from build123d import *

# Parameters (mm, degrees)
BOSS_EXTRUDE1_DEPTH = 2.5
FILLET1_R           = 6
FILLET2_R           = 1.5
SKETCH3_R           = 0.9999999999999983
CUT_EXTRUDE1_DEPTH  = 3.5
BOSS_EXTRUDE2_DEPTH = 2.6
SKETCH5_R           = 2.9999999999999947
CUT_EXTRUDE2_DEPTH  = 406.0937861882827
CUT_EXTRUDE3_DEPTH  = 3
FILLET3_R           = 6


with BuildPart() as part:
    # Sketch2 → Boss-Extrude1 (new body)
    with BuildSketch(Plane.XY.offset(10)):
        Polygon((-326.0372348081085, 240.3636560028167), (-313.73723480810855, 240.3636560028167), (-313.7372348081085, 216.3636560028167), (-326.0372348081085, 216.3636560028167), align=None)
    extrude(amount=BOSS_EXTRUDE1_DEPTH)

    # Fillet1
    fillet1_edges = [part.edges().sort_by_distance(p)[0] for p in [
        (-313.7372348081085, 216.3636560028167, 11.25),
        (-326.0372348081085, 216.3636560028167, 11.25),
    ]]
    fillet(fillet1_edges, radius=FILLET1_R)

    # Fillet2
    fillet2_edges = [part.edges().sort_by_distance(p)[0] for p in [
        (-326.0372348081085, 240.3636560028167, 11.25),
        (-313.73723480810855, 240.3636560028167, 11.25),
    ]]
    fillet(fillet2_edges, radius=FILLET2_R)

    # Sketch3 → Cut-Extrude1 (cut)
    with BuildSketch(Plane.XY.offset(12.5)):
        with Locations((-324.0490905957561, 237.3636560028167)):
            Circle(SKETCH3_R)
        with Locations((-315.94909059575616, 237.3636560028167)):
            Circle(SKETCH3_R)
    extrude(amount=-CUT_EXTRUDE1_DEPTH, mode=Mode.SUBTRACT)

    # Sketch4 → Boss-Extrude2 (add)
    with BuildSketch(Plane.XY.offset(12.5)):
        Polygon((-326.0372348081085, 233.42269782366114), (-313.7372348081087, 233.42269782366114), (-313.7372348081086, 216.42269782366117), (-326.0372348081085, 216.42269782366117), align=None)
    extrude(amount=BOSS_EXTRUDE2_DEPTH)

    # Sketch5 → Cut-Extrude2 (cut, through all)
    with BuildSketch(Plane.XY.offset(15.100000000000001)):
        with Locations((-319.88723480810853, 222.45389289856294)):
            Circle(SKETCH5_R)
    extrude(amount=-CUT_EXTRUDE2_DEPTH, mode=Mode.SUBTRACT)

    # Sketch6 → Cut-Extrude3 (cut)
    with BuildSketch(Plane.XY.offset(15.100000000000001)):
        with BuildLine():
            Line((-322.2509023799276, 231.87527778635172), (-317.6775841933858, 231.916179418332))
            Line((-317.6775841933858, 231.916179418332), (-317.06574253676285, 221.43449044480062))
            ThreePointArc((-317.06574253676285, 221.43449044480062), (-320.0096946123076, 219.21611603523496), (-322.9124096628873, 221.4881820948509))
            Line((-322.9124096628873, 221.4881820948509), (-322.2509023799276, 231.87527778635172))
        make_face()
    extrude(amount=-CUT_EXTRUDE3_DEPTH, mode=Mode.SUBTRACT)

    # Fillet3
    # the kernel refuses this fillet: 6 mm, written as the material it takes off along each edge
    with BuildSketch(Plane(origin=(-326.0372348081085, 216.42269782366117, -2.5000000000000018), x_dir=(1, 0, 0), z_dir=(0, 0, 1))) as fillet3_piece_1_section:
        with BuildLine():
            CenterArc((FILLET3_R, FILLET3_R), FILLET3_R, 180, 90)
            Line((0, FILLET3_R), (0, 0))
            Line((0, 0), (FILLET3_R, 0))
        make_face()
    fillet3_piece_1 = extrude(amount=32.6, mode=Mode.PRIVATE)
    fillet3_piece_1 = fillet3_piece_1 - Plane(origin=(-320.0372348081085, 222.3636560028167, 11.24999999999967), x_dir=(0, -1, 0), z_dir=(0, 0, 1)) * Cylinder(6, 90, mode=Mode.PRIVATE)
    add(fillet3_piece_1, mode=Mode.SUBTRACT)
    with BuildSketch(Plane(origin=(-326.0372348081085, 216.42269782366117, 12.5), x_dir=(1, 0, 0), z_dir=(0, 0, 1))) as fillet3_piece_2:
        with BuildLine():
            CenterArc((FILLET3_R, FILLET3_R), FILLET3_R, 180, 90)
            Line((0, FILLET3_R), (0, 0))
            Line((0, 0), (FILLET3_R, 0))
        make_face()
    extrude(amount=17.6, mode=Mode.SUBTRACT)
    with BuildSketch(Plane(origin=(-313.7372348081085, 216.42269782366117, -2.5000000000000018), x_dir=(0, 1, 0), z_dir=(0, 0, 1))) as fillet3_piece_3_section:
        with BuildLine():
            CenterArc((FILLET3_R, FILLET3_R), FILLET3_R, 180, 90)
            Line((0, FILLET3_R), (0, 0))
            Line((0, 0), (FILLET3_R, 0))
        make_face()
    fillet3_piece_3 = extrude(amount=32.6, mode=Mode.PRIVATE)
    fillet3_piece_3 = fillet3_piece_3 - Plane(origin=(-319.7372348081085, 222.3636560028167, 11.250000000000943), x_dir=(1, 2.37e-15, 0), z_dir=(0, 0, 1)) * Cylinder(6, 90, mode=Mode.PRIVATE)
    add(fillet3_piece_3, mode=Mode.SUBTRACT)
    with BuildSketch(Plane(origin=(-313.7372348081086, 216.42269782366117, 12.5), x_dir=(1.895e-14, 1, 0), z_dir=(0, 0, 1))) as fillet3_piece_4:
        with BuildLine():
            CenterArc((FILLET3_R, FILLET3_R), FILLET3_R, 180, 90.00000000000108)
            Line((-1.1369e-13, FILLET3_R), (0, 0))
            Line((0, 0), (FILLET3_R, 0))
        make_face()
    extrude(amount=17.6, mode=Mode.SUBTRACT)


solid = part.part
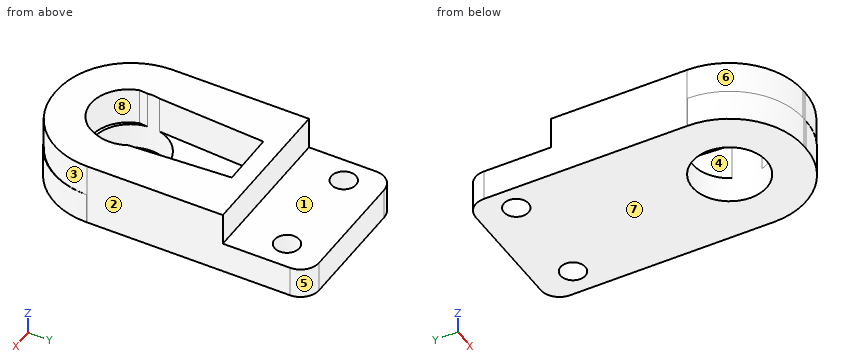
Input: part model. Units: mm. Frame: model coordinates. Face numbers are marked on the shaded views. A direction names the side the tool comes from. Coordinates: 2 decimals unless noted, no trailing zeros. Loops run counter-clockwise (first coordinate to the right, second up) from the corner with the lowest first, then second, coordinate; pieces in that order, holes last. Notation, with made-up numbers: (-33.5, 55.5) -> (-12.5, 55.5) arc R19 ccw to (-12.5, 79.5) -> close; hole circle Ø8 at (79.5, 71.25). An arc over 180 degrees is marked (long way). Write item = value, one per line. Start each with the question number.
Item 1: Cut plane A-A, the plane x = -321. Return loops of the section in (y, z), plus the area to 3 significant figures.
Item 2: Mould query, pull axis Y, two halves, no side actions, for the marked faces 5, 6, 7 and 8. Classes: pulls with the +Y half, pulls with the -Y half, needs draft (parallel to the pull), parting line crosses it, or undercut.
Item 3: Cut plane D-D, the plane z = 10.65. Count the separate pieces of the cut face and the enclosed holes in it, plus the area to 3 significant figures.
Item 4: Cut plane B-B, the plane z = 13.25. Return loops of the section in (x, y).
Item 5: First-contact query: P1, Ø1.5, axis at x = -320.5, y = 221, coming from the +Z side; P2, Ø4, axis at x = -317.5, y = 237, coming from the +Z side. Flat tips, straight axial feed; report the tip coordinate or a pass-through.
Item 6: Cut plane C-C, the plane y = 224.5. Return loops of the section in (x, z), plus the area to 3 significant figures.
Item 7: Reachability of the marked faces 1, 2, 3 and 4 from +Z, -Z, +X, -X, +Y, -Y: full face, straight path, thin tool, end or side. Return the list, or none.
Item 8: Material intervals for line 1 (Z direction, x = -320, y = 237.5); line 2 (Z direction, x = -318.25, y = 228); line 3 (Y direction, x = -318.5, z = 10.25), sorted ascending.
Ans:
q1.outline = (216.44, 10) -> (219.67, 10) -> (219.67, 12.1) -> (219.39, 12.1) -> (219.39, 15.1) -> (216.5, 15.1) -> (216.5, 12.5) -> (216.44, 12.5) -> close; (225.24, 10) -> (240.36, 10) -> (240.36, 12.5) -> (233.42, 12.5) -> (233.42, 15.1) -> (231.89, 15.1) -> (231.89, 12.1) -> (225.24, 12.1) -> close
q1.area = 54.6 mm²
q2.face_5 = pulls with the +Y half
q2.face_6 = pulls with the -Y half
q2.face_7 = needs draft
q2.face_8 = undercut
q3.separate_pieces = 1
q3.enclosed_holes = 3
q3.area = 244 mm²
q4.outline = (-326.04, 222.42) arc R6 ccw to (-320.04, 216.42) -> (-319.74, 216.42) arc R6 ccw to (-313.74, 222.42) -> (-313.74, 233.42) -> (-326.04, 233.42) -> close; hole (-322.91, 221.49) arc R3.03 ccw to (-317.07, 221.43) arc R3 ccw to (-317.2, 223.79) -> (-317.68, 231.92) -> (-322.25, 231.88) -> (-322.81, 223.14) arc R3 ccw to (-322.87, 222.14) -> close
q5.P1 = through
q5.P2 = 12.5
q6.outline = (-326.04, 10) -> (-322.08, 10) -> (-322.08, 12.1) -> (-322.72, 12.1) -> (-322.72, 15.1) -> (-326.04, 15.1) -> close; (-317.69, 10) -> (-313.74, 10) -> (-313.74, 15.1) -> (-317.24, 15.1) -> (-317.24, 12.1) -> (-317.69, 12.1) -> close
q6.area = 37.1 mm²
q7.face_1 = +Z, +X, -X, +Y
q7.face_2 = +Z, -Z, +X, +Y, -Y
q7.face_3 = +Z, +X, -Y
q7.face_4 = +Z
q8.line_1 = 10 to 12.5
q8.line_2 = 10 to 12.1
q8.line_3 = 216.49 to 219.79, 225.11 to 240.36
